Part print with two shaded views. Sizes in mm from the minimum x, y, z corner. A direction names the side the tool comes from. Coordinates: 2 decimals unless noted, no trailing zeros. Loops run counter-clockwise (first coordinate to the right, second up) from the corner with the lowest first, then second, coordinate; pieces in that order, holes last. Notation, with made-up numbers: (2, 48.25) -> (41, 48.25) arc R8 ccw to (41, 54.25) -> close; hole circle Ø8 at (8.5, 67). An arc over 180 degrees is marked (long way). Return JSON: item names as keys, results as strings. Group by question number.
(1) Saw through at D-D on x = 42. Write the cut outline in (y, z), then the cut area to 3 significant figures.
(2) Saw through at A-A on x = 54. Write the cut outline in (y, z), then the cut area to 4 significant figures.
(3) Flat gauge pins, fed straight in: pin 1 Ø4.5 at (x, z) = (19, 30.5) entering from +Y; pin 2 Ø1 at (y, z) = (29.5, 6) entering from -X; pin 3 Ø12 at (x, y) = (29, 38.5) entering from -Z. Where does each tip first touch, or does it go through?
(4) Tool access for the marked faces 1, 2 and 3: list every direction of +Z, -Z, +X, -X, +Y, -Y with a clear straight run to the whole face (end or side of a thin tool).
(5) Probe L1, parallel to Y at x = 14.5, z = 32.5; L2, parallel to Y at x = 39, z = 2; L3, parallel to Z at x = 49.5, y = 32. List the from-to ranges inside material, lowest first.
(6) Saw through at C-C on y = 28. Write the cut outline in (x, z), then the cut area to 4 significant figures.
(7) Saw through at B-B on z = 4. Write the cut outline in (x, y).
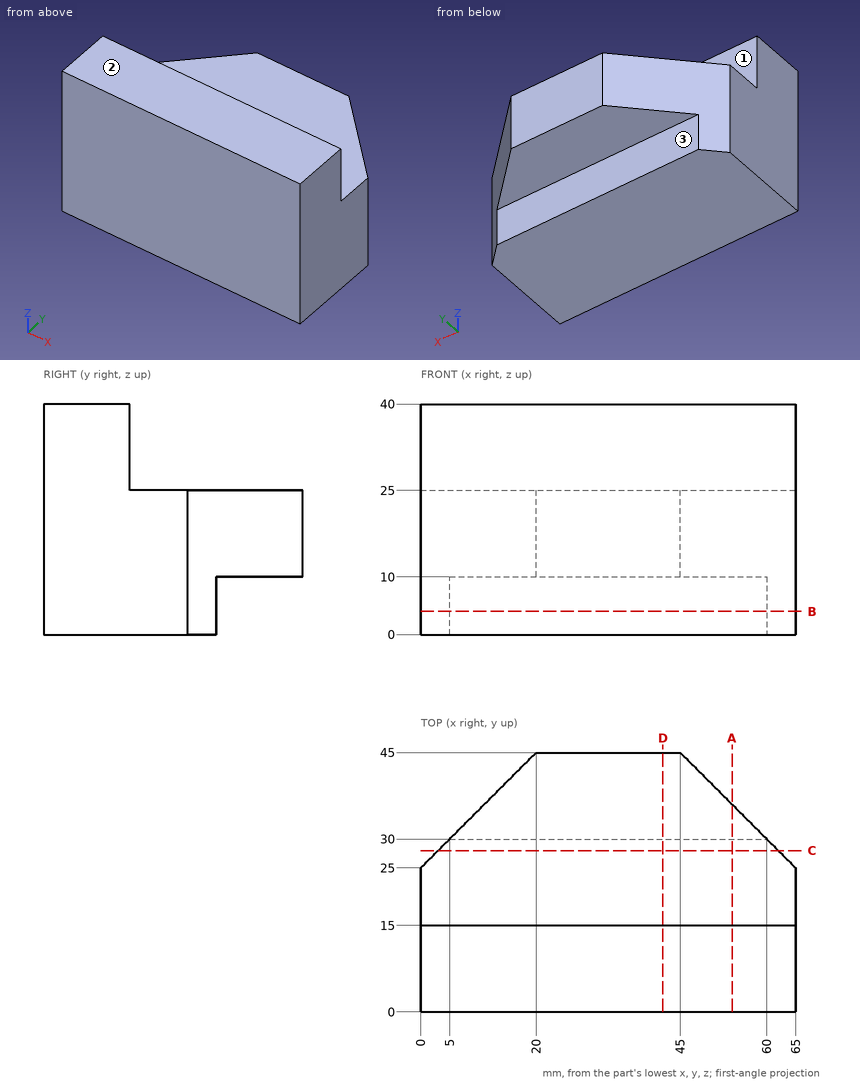
Geometry results:
{
 "1": {"outline": "(0, 0) -> (30, 0) -> (30, 10) -> (45, 10) -> (45, 25) -> (15, 25) -> (15, 40) -> (0, 40) -> close", "area": "1,200 mm²"},
 "2": {"outline": "(0, 0) -> (30, 0) -> (30, 10) -> (36, 10) -> (36, 25) -> (15, 25) -> (15, 40) -> (0, 40) -> close", "area": "1,065 mm²"},
 "3": {"pin 1": "y = 15", "pin 2": "x = 4", "pin 3": "z = 10"},
 "4": {"face 1": "+Z, +X, -X, +Y", "face 2": "+Z, +X, -X, +Y, -Y", "face 3": "-Z, +X, -X, +Y"},
 "5": {"L1": "0 to 15", "L2": "0 to 30", "L3": "10 to 25"},
 "6": {"outline": "(3, 0) -> (62, 0) -> (62, 25) -> (3, 25) -> close", "area": "1,475 mm²"},
 "7": {"outline": "(0, 0) -> (65, 0) -> (65, 25) -> (60, 30) -> (5, 30) -> (0, 25) -> close"}
}
